```python
from build123d import *

# Parameters (mm, degrees)
F0_R     = 3
F1_DEPTH = 10
F2_DEPTH = 1.5
F3_DEPTH = 5
F5_DEPTH = 2.5
F6_R     = 7.5
F7_DEPTH = 39.2


with BuildPart() as f1:
    # F0 (on Right) → F1 (new body)
    with BuildSketch(Plane.YZ):
        with BuildLine():
            ThreePointArc((20.61274, -13.2863032171), (31.1965214407, -0.8674840476), (35, 15))
            ThreePointArc((35, 15), (-15.6884798499, 46.2869237861), (-20.93552, -13.0482441933))
            Line((-20.93552, -13.0482441933), (-20.93552, -5))
            Line((-20.93552, -5), (20.61274, -5))
            Line((20.61274, -5), (20.61274, -13.2863032171))
        make_face()
        with BuildLine():
            ThreePointArc((-30, 25), (-18.2276824926, 25.8981970324), (-8, 20))
            ThreePointArc((-8, 20), (-22.6601045644, 6.3955399166), (-30, 25))
        make_face(mode=Mode.SUBTRACT)
        with BuildLine():
            ThreePointArc((8, 20), (18.2276824926, 25.8981970324), (30, 25))
            ThreePointArc((30, 25), (22.6601045644, 6.3955399166), (8, 20))
        make_face(mode=Mode.SUBTRACT)
        with BuildLine():
            ThreePointArc((20.61274, -13.2863032171), (-0.2005361733, -19.9994254988), (-20.93552, -13.0482441933))
            Line((-20.93552, -13.0482441933), (-20.93552, -35))
            Line((-20.93552, -35), (20.61274, -35))
            Line((20.61274, -35), (20.61274, -13.2863032171))
        make_face()
        with BuildLine():
            Line((-20.93552, -5), (-20.93552, -13.0482441933))
            ThreePointArc((-20.93552, -13.0482441933), (-0.2005361733, -19.9994254988), (20.61274, -13.2863032171))
            Line((20.61274, -13.2863032171), (20.61274, -5))
            Line((20.61274, -5), (-20.93552, -5))
        make_face()
        with BuildLine():
            ThreePointArc((-30, 25), (-22.6601045644, 6.3955399166), (-8, 20))
            ThreePointArc((-8, 20), (-18.2276824926, 25.8981970324), (-30, 25))
        make_face()
        with Locations((-13, 18)):
            Circle(F0_R, mode=Mode.SUBTRACT)
        with BuildLine():
            ThreePointArc((8, 20), (22.6601045644, 6.3955399166), (30, 25))
            ThreePointArc((30, 25), (18.2276824926, 25.8981970324), (8, 20))
        make_face()
        with Locations((13, 18)):
            Circle(F0_R, mode=Mode.SUBTRACT)
        with Locations((-13, 18)):
            Circle(F0_R)
        with Locations((13, 18)):
            Circle(F0_R)
    extrude(amount=F1_DEPTH)

    # F0 (on Right) → F2 (join)
    with BuildSketch(Plane.YZ):
        with BuildLine():
            ThreePointArc((-30, 25), (-22.6601045644, 6.3955399166), (-8, 20))
            ThreePointArc((-8, 20), (-18.2276824926, 25.8981970324), (-30, 25))
        make_face()
        with Locations((-13, 18)):
            Circle(F0_R, mode=Mode.SUBTRACT)
        with BuildLine():
            ThreePointArc((8, 20), (22.6601045644, 6.3955399166), (30, 25))
            ThreePointArc((30, 25), (18.2276824926, 25.8981970324), (8, 20))
        make_face()
        with Locations((13, 18)):
            Circle(F0_R, mode=Mode.SUBTRACT)
    extrude(amount=-F2_DEPTH)

    # F0 (on Right) → F3 (cut)
    with BuildSketch(Plane.YZ):
        with Locations((-13, 18)):
            Circle(F0_R)
        with Locations((13, 18)):
            Circle(F0_R)
    extrude(amount=F3_DEPTH, mode=Mode.SUBTRACT)

    # F4 (on face) → F5 (cut)
    with BuildSketch(Plane.YZ):
        with BuildLine():
            Line((-11, -12), (-16, -12))
            Line((-16, -12), (-16, -16.1287648325))
            ThreePointArc((-16, -16.1287648325), (-13.5406838246, -17.2746011836), (-11, -18.2264954517))
            Line((-11, -18.2264954517), (-11, -12))
        make_face()
        with BuildLine():
            Line((-7, -12), (-7, -19.292856399))
            ThreePointArc((-7, -19.292856399), (-4.5117191909, -19.7079874084), (-2, -19.9428104193))
            Line((-2, -19.9428104193), (-2, -12))
            Line((-2, -12), (-7, -12))
        make_face()
        with BuildLine():
            Line((2, -12), (2, -19.9428104193))
            ThreePointArc((2, -19.9428104193), (4.5117191909, -19.7079874084), (7, -19.292856399))
            Line((7, -19.292856399), (7, -12))
            Line((7, -12), (2, -12))
        make_face()
        with BuildLine():
            ThreePointArc((11, -18.2264954517), (13.5406838246, -17.2746011836), (16, -16.1287648325))
            Line((16, -16.1287648325), (16, -12))
            Line((16, -12), (11, -12))
            Line((11, -12), (11, -18.2264954517))
        make_face()
        with BuildLine():
            Line((16, -32), (16, -16.1287648325))
            ThreePointArc((16, -16.1287648325), (13.5406838246, -17.2746011836), (11, -18.2264954517))
            Line((11, -18.2264954517), (11, -32))
            Line((11, -32), (16, -32))
        make_face()
        with BuildLine():
            ThreePointArc((-11, -18.2264954517), (-13.5406838246, -17.2746011836), (-16, -16.1287648325))
            Line((-16, -16.1287648325), (-16, -32))
            Line((-16, -32), (-11, -32))
            Line((-11, -32), (-11, -18.2264954517))
        make_face()
        with BuildLine():
            ThreePointArc((7, -19.292856399), (4.5117191909, -19.7079874084), (2, -19.9428104193))
            Line((2, -19.9428104193), (2, -32))
            Line((2, -32), (7, -32))
            Line((7, -32), (7, -19.292856399))
        make_face()
        with BuildLine():
            ThreePointArc((-2, -19.9428104193), (-4.5117191909, -19.7079874084), (-7, -19.292856399))
            Line((-7, -19.292856399), (-7, -32))
            Line((-7, -32), (-2, -32))
            Line((-2, -32), (-2, -19.9428104193))
        make_face()
    extrude(amount=F5_DEPTH, mode=Mode.SUBTRACT)

    # F6 (on face) → F7 (cut)
    with BuildSketch(Plane.YZ):
        with Locations((0, 37.5)):
            Circle(F6_R)
    extrude(amount=F7_DEPTH, mode=Mode.SUBTRACT)


solid = f1.part
```
The listing builds one solid part. Answer for the finished solid, in the listing's coordinates (mm). A direction names the side the tool comes from. Give positions to 0.01 mm unless a question says otherwise; leave off trailing zeros. Order: outer loops, then holes, each group sorted by start corner. A loop starts at its lowest first (then second) coordinate and runs counter-clockwise, first axis right, second up.
Item 1: Given pin 1 Ø1 at (x, y) = (7.5, -23.5) entering from +Z; pin 2 Ø1.2 at (x, z) = (0.5, -25) entering from +Y; pin 3 Ø3 at (x, z) = (1.5, -23) entering from -Y, each flat-ended and moving along its own axis, determine where each tip first touches the part or whether it passes through.
From the geometry:
pin 1: stops at z = 41.38
pin 2: stops at y = 20.61
pin 3: stops at y = -20.94
Item 2: The part is cut by section D-D, the plane z = 13. Give the vertices of the cut face in (x, y).
From the geometry:
outline: (-1.5, -30.91) - (0, -30.91) - (0, -34.94) - (10, -34.94) - (10, 34.94) - (0, 34.94) - (0, 30.91) - (-1.5, 30.91) - (-1.5, 9.04) - (0, 9.04) - (0, -9.04) - (-1.5, -9.04) - close
Item 3: Which of the six approach directions +Z, -Z, +X, -X, +Y, -Y give full straight-line access (tool end or side, diameter ignored) to faces 1 (the face through (1, -5, -32)), 2 (the face through (5, 20.613, -24)), 3 (the face through (5, -20.936, -24)), 4 (the face through (-0.74, -18.06, 25.86))?
From the geometry:
face 1: -X
face 2: -Z, +X, -X, +Y
face 3: -Z, +X, -X, -Y
face 4: +Z, -X
Item 4: The part is cut by section C-C, the plane y = -13. Give the vertices of the cut face in (x, z).
From the geometry:
outline: (-1.5, 8.31) - (0, 8.31) - (0, -12) - (2.5, -12) - (2.5, -32) - (0, -32) - (0, -35) - (10, -35) - (10, 47.5) - (0, 47.5) - (0, 23.91) - (-1.5, 23.91) - (-1.5, 21) - (5, 21) - (5, 15) - (-1.5, 15) - close
Item 5: Find the intervals of material crossed by probe 1 along Y at (x, z) = (2, -27); probe 2 along Z at (x, y) = (5, 0); probe 3 along Z at (x, y) = (-0.65, -13), in increasing order.
From the geometry:
probe 1: y = -20.94 to -16, -11 to -7, -2 to 2, 7 to 11, 16 to 20.61
probe 2: z = -35 to 30, 45 to 50
probe 3: z = 8.31 to 15, 21 to 23.91
Item 6: The part is cut by section B-B, the plane z = -22.5. Give the vertices of the cut face in (x, y).
From the geometry:
outline: (0, -20.94) - (10, -20.94) - (10, 20.61) - (0, 20.61) - (0, 16) - (2.5, 16) - (2.5, 11) - (0, 11) - (0, 7) - (2.5, 7) - (2.5, 2) - (0, 2) - (0, -2) - (2.5, -2) - (2.5, -7) - (0, -7) - (0, -11) - (2.5, -11) - (2.5, -16) - (0, -16) - close
Item 7: The part is cut by section A-A, the plane y = 0. Give the vertices of the cut face in (x, z), and give its area (3 significant figures).
From the geometry:
outline: (0, -35) - (10, -35) - (10, 30) - (0, 30) - close; (0, 45) - (10, 45) - (10, 50) - (0, 50) - close
area: 700 mm2
Item 8: For a pull along Z with two mould halves and no side action, classify faces 5 (the face through (-1.5, 20, 16)), 6 (the face through (2.5, 13, -22)), 7 (the face through (-0.74, 22.338, 6.327)) as pulls with the +Z half, pulls with the -Z half, needs draft (parallel to the pull), parting line crosses it, or undercut.
From the geometry:
face 5: needs draft
face 6: undercut
face 7: parting line crosses it
